Geometry check sheet. Reference: the model listing, model coordinates, mm. A direction names the side the tool comes from. Coordinates: 2 decimals unless noted, no trailing zeros. Order: outer loops, then holes, each group sorted by start corner. A loop starts at its lowest first (then second) coordinate and runs counter-clockwise, first axis right, second up. Notation, with made-up numbers: (36, 9) - (56, 9) arc R17 ccw to (56, 35) - close; hole circle Ø7 at (-20.5, -19). An arc over 180 degrees is marked (long way). Put each result on its own line as item: value.
from build123d import *

# Parameters (mm, degrees)
SKETCH1_W              = 450
SKETCH1_H              = 450
BOSS_EXTRUDE1_DEPTH    = 10
SKETCH2_W              = 8.1
SKETCH2_H              = 27
SKETCH2_W_2            = 13.1
SKETCH2_H_2            = 6.8
CUT_EXTRUDE1_DEPTH     = 637.474665639
LPATTERN1_COUNT        = 3
LPATTERN1_PITCH        = 100
LPATTERN1_COL_COUNT    = 3
LPATTERN1_COL_PITCH    = 100
SKETCH3_W              = 70
SKETCH3_H              = 9
BOSS_EXTRUDE2_DEPTH    = 10
FILLET1_R              = 2.5
LPATTERN2_COUNT        = 4
LPATTERN2_PITCH        = 100
FILLET1_OF_LPATTERN2_R = 2.5
SKETCH4_W              = 390
SKETCH4_H              = 390
SKETCH4_W_2            = 60
SKETCH4_H_2            = 200
CUT_EXTRUDE2_DEPTH     = 637.474665639
CUT_EXTRUDE3_DEPTH     = 515.878626474
FILLET2_R              = 10
FILLET3_R              = 30


with BuildPart() as part:
    # Sketch1 → Boss-Extrude1 (new body)
    with BuildSketch(Plane(origin=(0, 0, 0), x_dir=(1, 0, 0), z_dir=(0, 1, 0))):
        with Locations((225, 225)):
            Rectangle(SKETCH1_W, SKETCH1_H)
    extrude(amount=BOSS_EXTRUDE1_DEPTH)

    # Sketch2 → Cut-Extrude1 (cut, through all)
    with BuildSketch(Plane(origin=(0, 10, 0), x_dir=(1, 0, 0), z_dir=(0, 1, 0))):
        with Locations((225, 3.5)):
            Rectangle(SKETCH2_W, SKETCH2_H)
        with Locations((225, 10)):
            Rectangle(SKETCH2_W_2, SKETCH2_H_2)
    cut_extrude1 = extrude(amount=-CUT_EXTRUDE1_DEPTH, mode=Mode.SUBTRACT)

    # LPattern1: Cut-Extrude1 ×3
    with Locations(*[(-i * LPATTERN1_PITCH, 0, 0) for i in range(1, LPATTERN1_COUNT)]):
        add(cut_extrude1, mode=Mode.SUBTRACT)

    # LPattern1 col: Cut-Extrude1 ×3
    with Locations(*[(i * LPATTERN1_COL_PITCH, 0, 0) for i in range(1, LPATTERN1_COL_COUNT)]):
        add(cut_extrude1, mode=Mode.SUBTRACT)

    # Sketch3 → Boss-Extrude2 (add)
    with BuildSketch(Plane(origin=(0, 10, 0), x_dir=(1, 0, 0), z_dir=(0, 1, 0))):
        with Locations((75, -4.5)):
            Rectangle(SKETCH3_W, SKETCH3_H)
    boss_extrude2 = extrude(amount=-BOSS_EXTRUDE2_DEPTH)

    # Fillet1
    fillet1_edges = [part.edges().sort_by_distance(p)[0] for p in [
        (110, 5, 9),
        (40, 5, 9),
    ]]
    fillet(fillet1_edges, radius=FILLET1_R)

    # LPattern2: Boss-Extrude2 ×4
    with Locations(*[(i * LPATTERN2_PITCH, 0, 0) for i in range(1, LPATTERN2_COUNT)]):
        add(boss_extrude2)

    # Fillet1 of LPattern2
    fillet1_of_lpattern2_edges = [part.edges().sort_by_distance(p)[0] for p in [
        (210, 5, 9),
        (140, 5, 9),
        (310, 5, 9),
        (240, 5, 9),
        (410, 5, 9),
        (340, 5, 9),
    ]]
    fillet(fillet1_of_lpattern2_edges, radius=FILLET1_OF_LPATTERN2_R)

    # Sketch4 → Cut-Extrude2 (cut, through all)
    with BuildSketch(Plane(origin=(0, 10, 0), x_dir=(1, 0, 0), z_dir=(0, 1, 0))):
        with Locations((255, 255)):
            Rectangle(SKETCH4_W, SKETCH4_H)
        with Locations((30, 350)):
            Rectangle(SKETCH4_W_2, SKETCH4_H_2)
    extrude(amount=-CUT_EXTRUDE2_DEPTH, mode=Mode.SUBTRACT)

    # Sketch5 → Cut-Extrude3 (cut, through all)
    with BuildSketch(Plane(origin=(0, 10, 0), x_dir=(1, 0, 0), z_dir=(0, 1, 0))):
        with BuildLine():
            Line((55, 40.5), (95, 40.5))
            ThreePointArc((95, 40.5), (110, 25.5), (95, 10.5))
            Line((95, 10.5), (55, 10.5))
            ThreePointArc((55, 10.5), (40, 25.5), (55, 40.5))
        make_face()
        with BuildLine():
            Line((155, 40.5), (195, 40.5))
            ThreePointArc((195, 40.5), (210, 25.5), (195, 10.5))
            Line((195, 10.5), (155, 10.5))
            ThreePointArc((155, 10.5), (140, 25.5), (155, 40.5))
        make_face()
        with BuildLine():
            Line((255, 40.5), (295, 40.5))
            ThreePointArc((295, 40.5), (310, 25.5), (295, 10.5))
            Line((295, 10.5), (255, 10.5))
            ThreePointArc((255, 10.5), (240, 25.5), (255, 40.5))
        make_face()
        with BuildLine():
            Line((355, 40.5), (395, 40.5))
            ThreePointArc((395, 40.5), (410, 25.5), (395, 10.5))
            Line((395, 10.5), (355, 10.5))
            ThreePointArc((355, 10.5), (340, 25.5), (355, 40.5))
        make_face()
        with BuildLine():
            Line((15, 55), (15, 95))
            ThreePointArc((15, 95), (30, 110), (45, 95))
            Line((45, 95), (45, 55))
            ThreePointArc((45, 55), (30, 40), (15, 55))
        make_face()
        with BuildLine():
            Line((45, 195), (45, 155))
            ThreePointArc((45, 155), (30, 140), (15, 155))
            Line((15, 155), (15, 195))
            ThreePointArc((15, 195), (30, 210), (45, 195))
        make_face()
    extrude(amount=-CUT_EXTRUDE3_DEPTH, mode=Mode.SUBTRACT)

    # Fillet2
    fillet2_edges = [part.edges().sort_by_distance(p)[0] for p in [
        (0, 5, -250),
        (450, 5, 0),
        (0, 5, 0),
    ]]
    fillet(fillet2_edges, radius=FILLET2_R)

    # Fillet3
    fillet3_edges = [part.edges().sort_by_distance(p)[0] for p in [
        (450, 5, -60),
        (60, 5, -60),
        (60, 5, -250),
    ]]
    fillet(fillet3_edges, radius=FILLET3_R)


solid = part.part
Q1. Section check D-D on y = 3.5. State how many separate pieces and enclosed holes the cut face has, then the cut area to 3 significant figures.
Answer block:
separate pieces: 1
enclosed holes: 6
area: 28,400 mm^2
Q2. Depth check by flat-ended pin: pin 1 Ø4 at (x, y) = (123.5, 5) entering from +Z; pin 2 Ø5 at (x, y) = (381.5, 6.5) entering from -Z; pin 3 Ø0.8 at (x, y) = (29.5, 7) entering from +Z. Enter the tip coordinate at first touch or a pass-through.
Answer block:
pin 1: stops at z = -17
pin 2: stops at z = -60
pin 3: stops at z = 0
Q3. Access from +Z, -Z, +X, -X, +Y, -Y to the whole of each face (thin tool, end or side, straight path). Record for faces 5 (the flat face through (60, 5, -154)), 6 (the cylindrical face through (30, 5, -40)), 7 (the flat face through (15, 5, 0)), 8 (the flat face through (157, 0, -54)), 9 (the flat face through (425, 5, -17)).
Answer block:
face 5: -Z, +X, +Y, -Y
face 6: +Y, -Y
face 7: +Z, -X, +Y, -Y
face 8: +Z, -Z, +X, -X, -Y
face 9: +Z, +Y, -Y
Q4. Section check C-C on z = -81. Record the boundary of the cut face in (x, y).
Answer block:
outline: (0, 0) - (15, 0) - (15, 10) - (0, 10) - close; (45, 0) - (61.38, 0) - (61.38, 10) - (45, 10) - close
Q5. Section check B-B on x = 184. Record the boundary of the cut face in (y, z), then the cut area to 3 significant figures.
Answer block:
outline: (0, -60) - (10, -60) - (10, -40.5) - (0, -40.5) - close; (0, -10.5) - (10, -10.5) - (10, 9) - (0, 9) - close
area: 390 mm^2
Q6. Section check A-A on z = -25.5. Record the boundary of the cut face in (x, y).
Answer block:
outline: (0, 0) - (40, 0) - (40, 10) - (0, 10) - close; (110, 0) - (140, 0) - (140, 10) - (110, 10) - close; (210, 0) - (240, 0) - (240, 10) - (210, 10) - close; (310, 0) - (340, 0) - (340, 10) - (310, 10) - close; (410, 0) - (450, 0) - (450, 10) - (410, 10) - close
Q7. Thickness scan on L1, parallel to Z at x = 258.5, y = 6; L2, parallel to X at y = 1.25, z = -183; L3, parallel to Z at x = 88, y = 3.5. Record the ranges inside material, lowest first. Write a range as [from, to].
Answer block:
L1: z = [-60, -40.5], [-10.5, 9]
L2: x = [0, 15], [45, 60]
L3: z = [-60.07, -40.5], [-10.5, 9]
Q8. Draft check along X on faces 1 (the cylindrical face through (40.004, 5.07, -25.17)), 2 (the flat face through (225, 5, -17)), 3 (the flat face through (157, 10, -54)), 4 (the cylindrical face through (440.979, 4.93, -51.445)). Enter one of: pulls with the +X half, pulls with the -X half, needs draft (parallel to the pull), parting line crosses it, or undercut.
Answer block:
face 1: undercut
face 2: undercut
face 3: needs draft
face 4: pulls with the +X half
